CAD build for the part. Positions are in the model's coordinates, mm. A direction names the side the tool comes from. Give positions to 0.01 mm unless a question says otherwise; leave off trailing zeros. Order: outer loops, then holes, each group sorted by start corner. A loop starts at its lowest first (then second) coordinate and runs counter-clockwise, first axis right, second up.
```python
from build123d import *

# Parameters (mm, degrees)
ESQUISSE2_W             = 20.5
ESQUISSE2_H             = 20.4
BOSS_EXTRU_1_DEPTH      = 4
ESQUISSE3_R             = 1.5
ESQUISSE3_R_2           = 0.75
ENL_V_MAT_EXTRU_1_DEPTH = 4
ESQUISSE4_W             = 2.2
ESQUISSE4_H             = 3
ESQUISSE4_W_2           = 2
ESQUISSE4_H_2           = 2.5
BOSS_EXTRU_2_DEPTH      = 1


with BuildPart() as part:
    # Esquisse2 → Boss.-Extru.1 (new body)
    with BuildSketch(Plane.XY):
        with Locations((10.25, 10.2)):
            Rectangle(ESQUISSE2_W, ESQUISSE2_H)
    extrude(amount=-BOSS_EXTRU_1_DEPTH)

    # Esquisse3 → Enlèv. mat.-Extru.1 (cut)
    with BuildSketch(Plane.XY):
        with Locations((2.5, 17.9)):
            Circle(ESQUISSE3_R)
        with Locations((18, 17.9)):
            Circle(ESQUISSE3_R)
        with Locations((2.63, 2)):
            Circle(ESQUISSE3_R_2)
        with Locations((5.17, 2)):
            Circle(ESQUISSE3_R_2)
        with Locations((7.71, 2)):
            Circle(ESQUISSE3_R_2)
        with Locations((10.25, 2)):
            Circle(ESQUISSE3_R_2)
        with Locations((12.79, 2)):
            Circle(ESQUISSE3_R_2)
        with Locations((15.33, 2)):
            Circle(ESQUISSE3_R_2)
        with Locations((17.87, 2)):
            Circle(ESQUISSE3_R_2)
    extrude(amount=-ENL_V_MAT_EXTRU_1_DEPTH, mode=Mode.SUBTRACT)

    # Esquisse4 → Boss.-Extru.2 (add)
    with BuildSketch(Plane.XY):
        with Locations((7.2, 10.3)):
            Rectangle(ESQUISSE4_W, ESQUISSE4_H)
        with Locations((10.5, 10.05)):
            Rectangle(ESQUISSE4_W_2, ESQUISSE4_H_2)
    extrude(amount=BOSS_EXTRU_2_DEPTH)


solid = part.part
```
Item 1: Slice it at B-B (y = 2). State how many separate pieces and enclosed holes the cut face has, and give its area (3 significant figures).
Item 2: Two-plate mould, pull along X, no slides. Class faces 6 (the face through (10, 10, 1)), 7 (the face through (3.345, 2.225, -1.972)), 8 (the face through (5.885, 2.225, -1.972)), 9 (the face through (6.1, 10.3, 0.5)): released by +X, released by -X, zero draft, split by the parting line, or undercut.
Item 3: Drop flat-ended pins along their axis: pin 1 Ø0.8 at (y, z) = (10.5, 0.5) entering from -X; pin 2 Ø0.5 at (x, z) = (11, 0.5) entering from +Y; pin 3 Ø2 at (x, y) = (7.71, 2) entering from +Z; pin 4 Ø1.4 at (x, y) = (5.17, 2) entering from +Z. Give the stop position or say it passes through.
Item 4: Slice it at D-D (y = 9.75). Give the cut face in (x, z).
Item 5: Wall check: L1, parallel to Y at x = 2.63, z = -2.8; L2, parallel to Y at x = 2.25, z = -0.8; L3, parallel to Z at x = 7.25, y = 13.75. Give the ranges that are in metal, low to high.
Item 6: Slice it at A-A (x = 10.25). Give the cut face in (y, z).
Item 7: Tool access for faces 1 (the face through (9.5, 10, 0.5)), 2 (the face through (10, 10, -4)), 3 (the face through (7.2, 11.8, 0.5)), 4 (the face through (7.2, 8.8, 0.5)), 5 (the face through (11.5, 10, 0.5)): list every direction of +Z, -Z, +X, -X, +Y, -Y with a clear straight run to the whole face (end or side of a thin tool).
A:
1. separate pieces: 8
1. enclosed holes: 0
1. area: 40.0 mm2
2. face 6: zero draft
2. face 7: undercut
2. face 8: undercut
2. face 9: released by -X
3. pin 1: stops at x = 6.1
3. pin 2: stops at y = 11.3
3. pin 3: stops at z = 0
3. pin 4: passes through
4. outline: (0, -4) - (20.5, -4) - (20.5, 0) - (11.5, 0) - (11.5, 1) - (9.5, 1) - (9.5, 0) - (8.3, 0) - (8.3, 1) - (6.1, 1) - (6.1, 0) - (0, 0) - close
5. L1: y = 0 to 1.25, 2.75 to 16.41, 19.39 to 20.4
5. L2: y = 0 to 1.35, 2.65 to 16.42, 19.38 to 20.4
5. L3: z = -4 to 0
6. outline: (0, -4) - (1.25, -4) - (1.25, 0) - (0, 0) - close; (2.75, -4) - (20.4, -4) - (20.4, 0) - (11.3, 0) - (11.3, 1) - (8.8, 1) - (8.8, 0) - (2.75, 0) - close
7. face 1: +Z, +Y, -Y
7. face 2: -Z, +X, -X, +Y, -Y
7. face 3: +Z, +X, -X, +Y
7. face 4: +Z, +X, -X, -Y
7. face 5: +Z, +X, +Y, -Y
